```python
from build123d import *

# Parameters (mm, degrees)
SKETCH1_R           = 2
SKETCH1_R_2         = 1.5
EXTRUDE1_DEPTH      = 3
CUT_EXTRUDE1_DEPTH  = 10
BOSS_EXTRUDE1_DEPTH = 3
CUT_EXTRUDE2_DEPTH  = 5


with BuildPart() as part:
    # Sketch1 → Extrude1 (new body)
    with BuildSketch(Plane.XY):
        with BuildLine():
            ThreePointArc((-26.085308936, -49.243272897), (-24.983078735, -55.562467556), (-18.568566007, -55.596511855))
            ThreePointArc((-18.568566007, -55.596511855), (9.955092257, -6.447651038), (9.831223687, 50.378348795))
            ThreePointArc((9.831223687, 50.378348795), (4.259504767, 53.557286163), (0.144535316, 48.6362374))
            ThreePointArc((0.144535316, 48.6362374), (0.489229737, -3.910438591), (-26.085308936, -49.243272897))
        make_face()
        with Locations((-21.755464684, -51.7437626)):
            Circle(SKETCH1_R, mode=Mode.SUBTRACT)
        with BuildLine():
            ThreePointArc((5.144535316, -3.1637626), (7.076357694, -5.681509932), (4.144339435, -6.895700301))
            ThreePointArc((4.144339435, -6.895700301), (3.212712938, -4.646015269), (5.144535316, -3.1637626))
        make_face(mode=Mode.SUBTRACT)
        with Locations((5.144535316, 48.6362374)):
            Circle(SKETCH1_R_2, mode=Mode.SUBTRACT)
    extrude(amount=EXTRUDE1_DEPTH)

    # Sketch3 → Cut-Extrude1 (cut)
    with BuildSketch(Plane(origin=(0, 0, 0), x_dir=(-1, 0, 0), z_dir=(0, 0, -1))):
        with BuildLine():
            ThreePointArc((26.085308936, -49.243272897), (16.272417408, -38.139391171), (8.225333931, -25.696181093))
            ThreePointArc((8.225333931, -25.696181093), (13.854681069, -38.186869472), (20.909608136, -49.931436277))
            ThreePointArc((20.909608136, -49.931436277), (22.829775371, -50.05679593), (23.755464684, -51.7437626))
            ThreePointArc((23.755464684, -51.7437626), (21.27804664, -53.685944881), (19.983392673, -50.816529735))
            ThreePointArc((19.983392673, -50.816529735), (8.408185994, -40.542939738), (-1.362976888, -28.540588427))
            ThreePointArc((-1.362976888, -28.540588427), (7.552683596, -42.842145312), (18.568566007, -55.596511855))
            ThreePointArc((18.568566007, -55.596511855), (24.983078735, -55.562467556), (26.085308936, -49.243272897))
        make_face()
    extrude(amount=-CUT_EXTRUDE1_DEPTH, mode=Mode.SUBTRACT)

    # Sketch3_3 → Boss-Extrude1 (add)
    with BuildSketch(Plane(origin=(0, 0, 0), x_dir=(-1, 0, 0), z_dir=(0, 0, -1))):
        with BuildLine():
            ThreePointArc((8.225333931, -25.696181093), (0.709764151, 9.885397236), (4.515866122, 46.052317111))
            ThreePointArc((4.515866122, 46.052317111), (-2.521867284, 58.28619141), (-14.783886482, 51.297610936))
            ThreePointArc((-14.783886482, 51.297610936), (-16.914814846, 9.892262753), (-1.362976888, -28.540588427))
            ThreePointArc((-1.362976888, -28.540588427), (-13.044605865, 10.119739731), (-9.831223687, 50.378348795))
            ThreePointArc((-9.831223687, 50.378348795), (-4.259504767, 53.557286163), (-0.144535316, 48.6362374))
            ThreePointArc((-0.144535316, 48.6362374), (-3.243862831, 10.649816422), (8.225333931, -25.696181093))
        make_face()
        with BuildLine():
            ThreePointArc((19.983392673, -50.816529735), (20.822206397, -50.767144538), (20.909608136, -49.931436277))
            ThreePointArc((20.909608136, -49.931436277), (20.37371395, -50.297814846), (19.983392673, -50.816529735))
        make_face()
    extrude(amount=-BOSS_EXTRUDE1_DEPTH)

    # Sketch4 → Cut-Extrude2 (cut)
    with BuildSketch(Plane(origin=(0, 0, 0), x_dir=(-1, 0, 0), z_dir=(0, 0, -1))):
        with BuildLine():
            ThreePointArc((-9.964210899, 49.966924168), (-13.222981584, 23.962412042), (-8.924214856, -1.890534442))
            ThreePointArc((-8.924214856, -1.890534442), (-6.34883687, -0.310963638), (-3.333762814, -0.503172193))
            ThreePointArc((-3.333762814, -0.503172193), (-4.204319589, 23.570760268), (-0.314334597, 47.344277255))
            ThreePointArc((-0.314334597, 47.344277255), (-6.455869332, 43.811260395), (-9.964210899, 49.966924168))
        make_face()
        with BuildLine():
            ThreePointArc((-5.849425706, -10.11382619), (-3.738208311, -9.961912697), (-1.879022525, -8.950109944))
            ThreePointArc((-1.879022525, -8.950109944), (0.268148473, -17.628892121), (3.046878131, -26.126554438))
            ThreePointArc((3.046878131, -26.126554438), (-1.805817512, -18.34494551), (-5.849425706, -10.11382619))
        make_face()
    extrude(amount=-CUT_EXTRUDE2_DEPTH, mode=Mode.SUBTRACT)


solid = part.part
```
The listing builds one solid part. Answer for the finished solid, in the listing's coordinates (mm). Coordinates: 2 decimals unless noted, no trailing zeros. Write each loop counter-clockwise with the first axis right and the second up, starting at its lowest first coordinate (ties: lowest second). Pieces come first, ordered by that corner, then holes. Notation, with made-up numbers: M 17,-10.5 L 33,-10.5 A19 cw 33,-1.5 Z; hole C 7.5,84 d6. An arc over 180 degrees is marked long. Use a Markdown table: item, result. Add a question column.
1. For a pull along Y with two mould halves and no side action, classify faces 1 (the cylindrical face through (4.225, 23.234, 1.479)), 2 (the flat face through (3, 8, 3)) as +Y half, -Y half, draft (parallel to the pull), parting line (faces both ways), or undercut.
2. Section B-B (z = 0.85) is taken. Give the vertices of the cut face in (x, y).
3. Section A-A (y = 37) is taken. Give the vertices of the cut face in (x, z).
4. Section D-D (x = -15) is taken. Give the vertices of the cut face in (y, z), plus the area to 3 significant figures.
5. Given P1, Ø3.5, axis at x = 5.14, y = -5.16, coming from the +Z side, flat-ended and moving along its own axis, determine where the tip first touches the part or whether it passes through.
6. Straight lines are drawn through the part: line 1 along X through (y, z) = (48, 1.8); line 2 along X through (y, z) = (-24, 1.35); line 3 along X through (y, z) = (-6, 0.1). For each, find the intervals that lie inside material, in ascending order. Write a range as [from, to].
7. Section C-C (y = 15) is taken. Give the vertices of the cut face in (x, z).
Data:
| question | item | result |
|---|---|---|
| 1 | face 1 | undercut |
| 1 | face 2 | draft |
| 2 | outline | M -20.91,-49.93 A0.65 ccw -19.98,-50.82 A95.87 ccw 14.78,51.3 A10 ccw -4.52,46.05 A116.66 cw Z; hole M -3.05,-26.13 A90.87 ccw 5.85,-10.11 A5 cw 1.88,-8.95 A121.66 cw Z; hole M 0.31,47.34 A121.66 cw 3.33,-0.5 A5 cw 8.92,-1.89 A90.87 ccw 9.96,49.97 A5 cw long Z; hole C 5.14,-5.16 d4; hole C 5.14,48.64 d3 |
| 3 | outline | M -2.48,0 L 2.6,0 L 2.6,3 L -2.48,3 Z; M 12.55,0 L 17.58,0 L 17.58,3 L 12.55,3 Z |
| 4 | outline | M -46.8,0 L -40.32,0 L -40.32,3 L -46.8,3 Z |
| 4 | area | 19.4 mm2 |
| 5 | P1 | passes through |
| 6 | line 1 | x = [-4.84, 3.79], [6.5, 10.1], [10.48, 15.63] |
| 6 | line 2 | x = [-7.59, -2.29], [-1.61, 4.3] |
| 6 | line 3 | x = [-2.63, 3.33], [6.96, 12.82] |
| 7 | outline | M -0.56,0 L 4.44,0 L 4.44,3 L -0.56,3 Z; M 12.6,0 L 17.63,0 L 17.63,3 L 12.6,3 Z |
